Design review of the part shown in the three views and the two pictorial views. Dimensions are in mm from the part's minimum x, y and z. Round coordinates to 2 decimals unless told otherwise and drop trailing zeros. Write each loop counter-clockwise with the first axis right and the second up, starting at its lowest first coordinate (ties: lowest second). Pieces come first, ordered by that corner, then holes. Notation, with made-up numbers: (-0.5, 58.25) - (23.5, 58.25) arc R34 cw to (23.5, 90.25) - close; hole circle Ø11 at (8, 31.25). An arc over 180 degrees is marked (long way). Use one line per item in the form item = value.
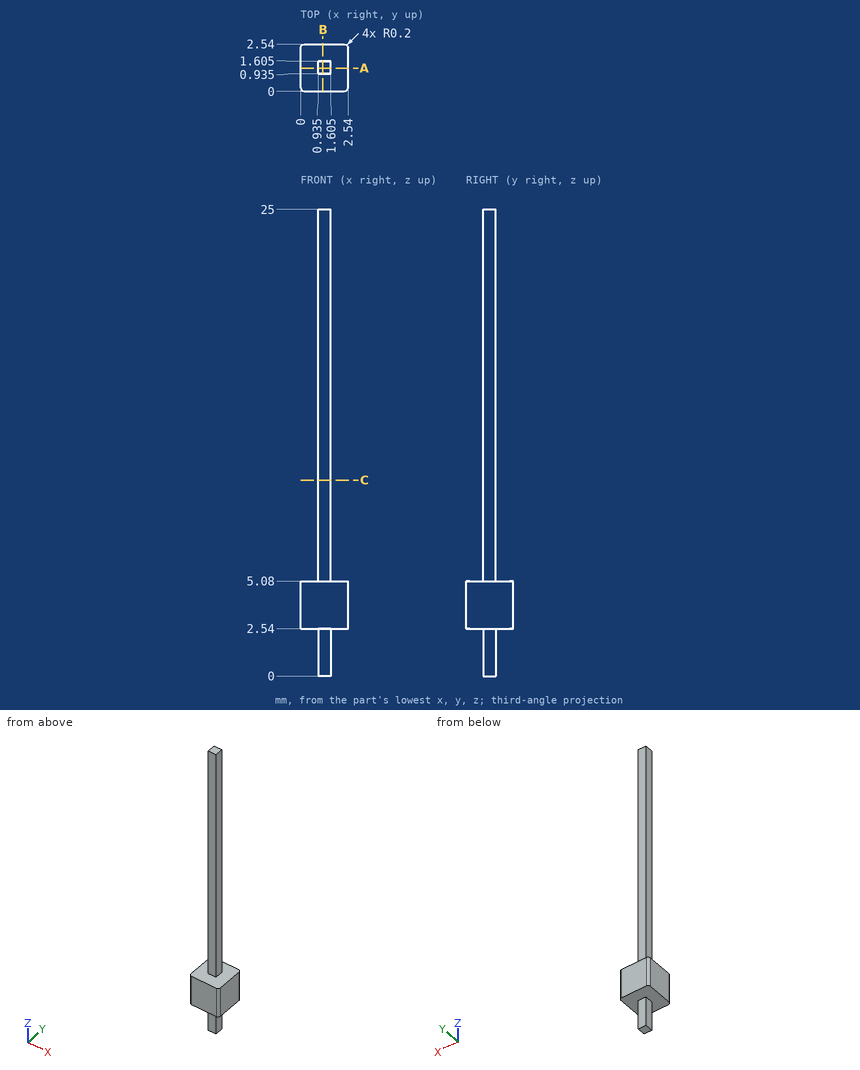
(1) Insertion check: P1, Ø0.8, axis at x = 1.5, y = 1.5, coming from the -Z side; P2, Ø0.5, axis at x = 1.5, z = 12.5, coming from the -Y side (3 decimals); P3, Ø1, axis at y = 1, z = 21.5, coming from the -X side (3 decimals); P4, Ø0.7, axis at y = 1, z = 19, coming from the +X side (3 decimals). Each pin has a flat end and moves straight along its axis. Give the tip position at first contact, or say it passes through.
Geometry results:
P1 = 0
P2 = 0.935
P3 = 0.935
P4 = 1.605
(2) To check wall thickness, follow L1, parallel to Z at x = 1.4, y = 2.4; L2, parallel to X at y = 1.1, z = 22.5 (3 decimals). State the ranges of each line that lie inside material, in increasing order.
Geometry results:
L1 = 2.54 to 5.08
L2 = 0.935 to 1.605
(3) Add section A-A on y = 1.25. Write out the cut boundary in (x, z) (3 decimals), then the cut area to 3 significant figures.
Geometry results:
outline = (0, 2.54) - (0.935, 2.54) - (0.935, 0) - (1.605, 0) - (1.605, 2.54) - (2.54, 2.54) - (2.54, 5.08) - (1.605, 5.08) - (1.605, 25) - (0.935, 25) - (0.935, 5.08) - (0, 5.08) - close
area = 21.5 mm2
(4) Add section C-C on z = 10.5. Write out the cut boundary in (x, y) (3 decimals), then the cut area to 3 significant figures.
Geometry results:
outline = (0.935, 0.935) - (1.605, 0.935) - (1.605, 1.605) - (0.935, 1.605) - close
area = 0.449 mm2
